Read the model definition and answer for the solid it produces. Units are mm, in the model's axes. Face numbers are marked on the shaded views. A direction names the side the tool comes from. Give positions to 0.01 mm unless a question says otherwise; leave off trailing zeros. Write each loop counter-clockwise with the first axis right and the second up, starting at its lowest first coordinate (ties: lowest second). Pieces come first, ordered by that corner, then holes. Notation, with made-up numbers: (-6, 47.25) -> (10, 47.25) arc R15 ccw to (10, 57.25) -> close; hole circle Ø11 at (-11, -35.75). An arc over 180 degrees is marked (long way). Use a Markdown table: item, result.
from build123d import *

# Parameters (mm, degrees)
SKETCH1_R           = 46
BOSS_EXTRUDE1_DEPTH = 3
SKETCH3_R           = 3.05
CUT_EXTRUDE2_DEPTH  = 1.1
CUT_EXTRUDE1_DEPTH  = 2.2
SKETCH4_R           = 7.5
BOSS_EXTRUDE2_DEPTH = 40
CHAMFER1_SIZE       = 6
SIZE_MEDICINE_REACH = 84.952
SKETCH5_W           = 10
SKETCH5_H           = 16
FILLET1_R           = 2


with BuildPart() as part:
    # Sketch1 → Boss-Extrude1 (new body)
    with BuildSketch(Plane.XY):
        with Locations((0, 8)):
            Circle(SKETCH1_R)
    extrude(amount=BOSS_EXTRUDE1_DEPTH)

    # Sketch3 → Cut-Extrude2 (cut)
    with BuildSketch(Plane(origin=(0, 0, 0), x_dir=(-1, 0, 0), z_dir=(0, 0, -1))):
        Circle(SKETCH3_R)
        with Locations(Location((0, 16, 0), (0, 0, 180))):
            Circle(SKETCH3_R)
    extrude(amount=-CUT_EXTRUDE2_DEPTH, mode=Mode.SUBTRACT)

    # Sketch2 → Cut-Extrude1 (cut)
    with BuildSketch(Plane(origin=(0, 0, 0), x_dir=(-1, 0, 0), z_dir=(0, 0, -1))):
        with BuildLine():
            Line((-7.95, 9.05), (-7.95, 6.95))
            ThreePointArc((-7.95, 6.95), (-9, 5.9), (-10.05, 6.95))
            Line((-10.05, 6.95), (-10.05, 9.05))
            ThreePointArc((-10.05, 9.05), (-9, 10.1), (-7.95, 9.05))
        make_face()
        with BuildLine():
            Line((7.95, 9.05), (7.95, 6.95))
            ThreePointArc((7.95, 6.95), (9, 5.9), (10.05, 6.95))
            Line((10.05, 6.95), (10.05, 9.05))
            ThreePointArc((10.05, 9.05), (9, 10.1), (7.95, 9.05))
        make_face()
    extrude(amount=-CUT_EXTRUDE1_DEPTH, mode=Mode.SUBTRACT)

    # Sketch4 → Boss-Extrude2 (add)
    with BuildSketch(Plane.XY.offset(3)):
        with Locations((0, 8)):
            Circle(SKETCH4_R)
    extrude(amount=BOSS_EXTRUDE2_DEPTH)

    # Chamfer1
    chamfer1_edges = [part.edges().sort_by_distance(p)[0] for p in [
        (-7.5, 8, 43),
    ]]
    chamfer(chamfer1_edges, length=CHAMFER1_SIZE)

    # Sketch5 → Size-Medicine (cut, up to next)
    with BuildSketch(Plane(origin=(0, 0, 0), x_dir=(-1, 0, 0), z_dir=(0, 0, -1)), mode=Mode.PRIVATE) as size_medicine_sk1:
        with Locations((41, 8)):
            Rectangle(SKETCH5_W, SKETCH5_H)
    size_medicine_tool1 = extrude(size_medicine_sk1.sketch, amount=-SIZE_MEDICINE_REACH, mode=Mode.PRIVATE) & part.part
    add(size_medicine_tool1.solids().sort_by_distance((-41, 8, 0))[0], mode=Mode.SUBTRACT)

    # Fillet1
    fillet1_edges = [part.edges().sort_by_distance(p)[0] for p in [
        (-45.299006612, 0, 1.5),
        (-45.299006612, 16, 1.5),
        (-36, 16, 1.5),
        (-36, 0, 1.5),
    ]]
    fillet(fillet1_edges, radius=FILLET1_R)


solid = part.part
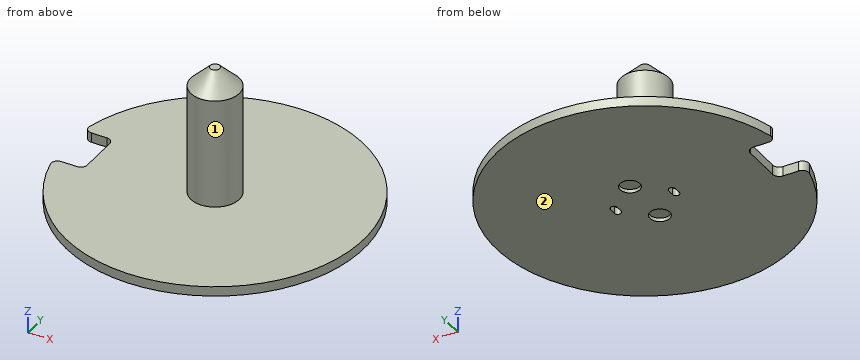
Item 1: A cutting plane is placed at C-C (y = 44). Give the vertices of the cut face in (x, z), then the cut area to 3 significant figures.
Return value:
| item | result |
|---|---|
| outline | (-28.64, 0) -> (28.64, 0) -> (28.64, 3) -> (-28.64, 3) -> close |
| area | 172 mm^2 |
Item 2: A cutting plane is placed at B-B (z = 16.5). Give the vertices of the cut face in (x, y), then the cut area to 3 significant figures.
Return value:
| item | result |
|---|---|
| outline | circle Ø15 at (0, 8) |
| area | 177 mm^2 |
Item 3: A tool of negligible diameter and unlimited length cuts with its end or side. For the marked faces 1 and 2, from which of +Z, -Z, +X, -X, +Y, -Y can it reach the whole face along a straight path? Write none if from no direction.
Return value:
| item | result |
|---|---|
| face 1 | +Z |
| face 2 | -Z, +X, -X, +Y, -Y |
Item 4: Each of these flat-tipped pins is pushed along its axis until it touches: P1, Ø5, axis at x = 0.5, y = 16.5, coming from the -Z side; P2, Ø3.5, axis at x = 0, y = 16, coming from the -Z side; P3, Ø1.5, axis at x = -41, z = 1, coming from the +Y side; P4, Ø0.9, axis at y = 9.5, z = 1.5, coming from the -X side. Where does it stop, or does it pass through?
Return value:
| item | result |
|---|---|
| P1 | z = 0 |
| P2 | z = 1.1 |
| P3 | y = 30.27 |
| P4 | x = -36 |
Item 5: A cutting plane is placed at A-A (x = 0). Give the vertices of the cut face in (y, z), then the cut area to 3 significant figures.
Return value:
| item | result |
|---|---|
| outline | (-38, 0) -> (-3.05, 0) -> (-3.05, 1.1) -> (3.05, 1.1) -> (3.05, 0) -> (12.95, 0) -> (12.95, 1.1) -> (19.05, 1.1) -> (19.05, 0) -> (54, 0) -> (54, 3) -> (15.5, 3) -> (15.5, 37) -> (9.5, 43) -> (6.5, 43) -> (0.5, 37) -> (0.5, 3) -> (-38, 3) -> close |
| area | 827 mm^2 |
Item 6: Straight lines are drawn through the part: line 1 along Y through (x, z) = (0, 0.7); line 2 along Y through (x, z) = (-0.5, 15); line 3 along Z through (x, y) = (-5.5, 24.5). For each, find the intervals that lie inside material, in ascending order. Write a range as [from, to].
Return value:
| item | result |
|---|---|
| line 1 | [-38, -3.05], [3.05, 12.95], [19.05, 54] |
| line 2 | [0.52, 15.48] |
| line 3 | [0, 3] |
Item 7: A cutting plane is placed at D-D (x = -32). Give the vertices of the cut face in (y, z).
Return value:
| item | result |
|---|---|
| outline | (-25.05, 0) -> (41.05, 0) -> (41.05, 3) -> (-25.05, 3) -> close |
